```python
from build123d import *

# Parameters (mm, degrees)
SKETCH12_R          = 10
BOSS_EXTRUDE2_DEPTH = 100
SKETCH13_R          = 10
BOSS_EXTRUDE3_DEPTH = 50
SHELL7_OUTLINE_R    = 7.7
SHELL7_DEPTH        = 100
SHELL7_START        = -1e-07
SHELL7_2_OUTLINE_R  = 7.7
SHELL7_2_DEPTH      = 50.0000001


with BuildPart() as part:
    # Sketch12 → Boss-Extrude2 (new body)
    with BuildSketch(Plane.XY):
        with Locations(Location((0, 0, 0), (0, 0, 180))):
            Circle(SKETCH12_R)
    extrude(amount=BOSS_EXTRUDE2_DEPTH)

    # Sketch13 → Boss-Extrude3 (add)
    with BuildSketch(Plane(origin=(0, 0, 0), x_dir=(0, 0, -1), z_dir=(1, 0, 0))):
        with Locations((-50, 0)):
            Circle(SKETCH13_R)
    extrude(amount=BOSS_EXTRUDE3_DEPTH)

    # Shell7: read off the stored shape, not the designer's step
    # Shell7 outline → Shell7 (cut)
    with BuildSketch(Plane.XY):
        Circle(SHELL7_OUTLINE_R)
    extrude(amount=SHELL7_DEPTH, mode=Mode.SUBTRACT)

    # Shell7 2 outline → Shell7 2 (cut)
    with BuildSketch(Plane.YZ.offset(SHELL7_START)):
        with Locations((0, 50)):
            Circle(SHELL7_2_OUTLINE_R)
    extrude(amount=SHELL7_2_DEPTH, mode=Mode.SUBTRACT)


solid = part.part
```
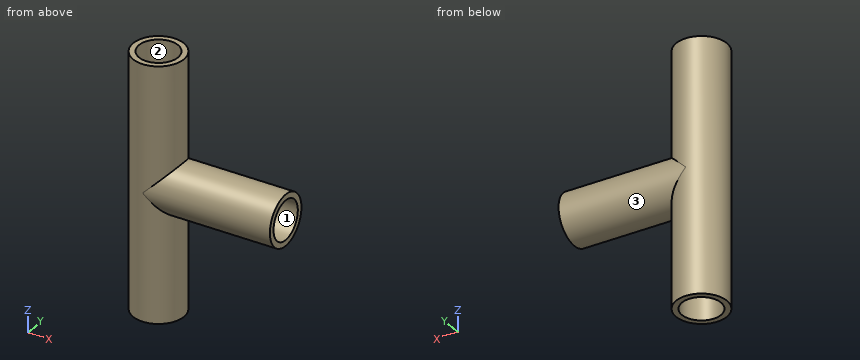
Design review of the part built by this model. Coordinates are the model's own, in mm. Face numbers are marked on the shaded views. Round coordinates to 2 decimals unless told otherwise and drop trailing zeros. Order: outer loops, then holes, each group sorted by start corner. A loop starts at its lowest first (then second) coordinate and runs counter-clockwise, first axis right, second up. Notation, with made-up numbers: (-33.5, 7.25) - (0.5, 7.25) arc R26 ccw to (0.5, 28.25) - close; hole circle Ø2 at (37, 72). An arc over 180 degrees is marked (long way). One line per question, with ' | ' between items.
Item 1: Take a section at D-D, the plane x = 19.5. Write out the cut boundary in (y, z), then the cut area to 3 significant figures.
Checks:
outline: circle Ø20 at (0, 50); hole circle Ø15.4 at (0, 50) | area: 128 mm²
Item 2: Wall thickness on line 1 (Y direction, x = 0, z = 26.5); line 2 (Z direction, x = 32, y = 0); line 3 (X direction, y = -3.5, z = 26): over which ranges is each line inside the solid? List them lowest first. Write a range as [from, to].
Checks:
line 1: [-10, -7.7], [7.7, 10] | line 2: [40, 42.3], [57.7, 60] | line 3: [-9.37, -6.86], [6.86, 9.37]
Item 3: For P1, Ø12, axis at y = 5.5, z = 70, coming from the +X side; P2, Ø8, axis at x = 31.5, y = -1, coming from the -Z side; P3, Ø4, axis at y = -5.5, z = 36, coming from the -X side, all flat-tipped, find the tip position at first contact; note any pin that passes through.
Checks:
P1: x = 10 | P2: z = 40 | P3: x = -9.37
Item 4: Take a section at A-A, the plane y = 0. Write out the cut boundary in (x, z).
Checks:
outline: (-10, 0) - (-7.7, 0) - (-7.7, 100) - (-10, 100) - close; (7.7, 0) - (10, 0) - (10, 40) - (50, 40) - (50, 42.3) - (7.7, 42.3) - close; (7.7, 57.7) - (50, 57.7) - (50, 60) - (10, 60) - (10, 100) - (7.7, 100) - close
Item 5: Draft analysis for pull direction Z (two halves, no side actions). For the marked faces 1, 2 and 3, state which applies: +Z half, -Z half, draft (parallel to the pull), parting line (faces both ways), or undercut.
Checks:
face 1: undercut | face 2: draft | face 3: parting line
Item 6: Take a section at C-C, the plane z = 80.5. Write out the cut boundary in (x, y).
Checks:
outline: circle Ø20 at (0, 0); hole circle Ø15.4 at (0, 0)
Item 7: Take a section at B-B, the plane z = 50. Write out the cut boundary in (x, y).
Checks:
outline: (0, -10) - (50, -10) - (50, -7.7) - (0, -7.7) arc R7.7 cw to (0, 7.7) - (50, 7.7) - (50, 10) - (0, 10) arc R10 ccw to start
